Build history of the part. All positions in model axes, mm. Round coordinates to 2 decimals unless told otherwise and drop trailing zeros. Order: outer loops, then holes, each group sorted by start corner. A loop starts at its lowest first (then second) coordinate and runs counter-clockwise, first axis right, second up. Notation, with made-up numbers: M -33.75,5.25 L 8.25,5.25 A15 cw 8.25,9.25 Z; hole C 41.25,51.25 d6. An arc over 180 degrees is marked long. One line per item, written item: value. Start each with the question number.
Item 1: Band-saw the part on C-C, the plane x = 1.4. Write the cut outline in (y, z), then the cut area to 3 significant figures.
Item 2: Probe L1, parallel to Z at x = 1.15, y = 0; L2, parallel to Z at x = 1.3, y = 12.5; L3, parallel to Y at x = 2.15, z = 9.5. List the from-to ranges inside material, lowest first.
Item 3: Band-saw the part on A-A, the plane z = 0. Write the cut outline in (x, y), then the cut area to 3 significant figures.
Item 4: Pin check, flat tip, straight feed: pin 1 (1.5 mm diameter, centred on x = 0.5, z = 20.5, fed in from -Y). Stop position of the tip, or through.
Autodesk Inventor part; units mm, degrees
ref_plane "SW_HW_XY" through (-8.6667, 0, 0) normal (1, 0, 0) x (0, 0, -1)
ref_plane "SW_HW_YZ" through (-8.6667, 0, 0) normal (0, 0, -1) x (0, 1, 0)
ref_plane "SW_HW_ZX" through (-8.6667, 0, 0) normal (0, 1, 0) x (1, 0, 0)
sketch "Sketch_1" plane through (0, 0, 0) normal (0, 0, 1) x (1, 0, 0)
  line L0 (3.3333, 0) -> (0, 0)
  arc A0 (0, 20.8756) -> (0, 23.6244) centre (-2.6667, 22.25) ccw
  line L1 (0, 20.8756) -> (0, 18.1)
  arc A1 (0, 18.1) -> (0.6, 17.5) centre (0.6, 18.1) ccw
  line L2 (0.6, 17.5) -> (2.7333, 17.5)
  arc A2 (2.7333, 17.5) -> (3.3333, 18.1) centre (2.7333, 18.1) ccw
  line L3 (3.3333, 18.1) -> (3.3333, 25.4)
  arc A3 (3.3333, 25.4) -> (2.7333, 26) centre (2.7333, 25.4) ccw
  line L4 (2.7333, 26) -> (0.6, 26)
  arc A4 (0.6, 26) -> (0, 25.4) centre (0.6, 25.4) ccw
  line L5 (0, 25.4) -> (0, 23.6244)
revolve "Revolution1" add sketch "Sketch_1" angle 360 about axis through (3.3333, 0, 0) along (1, 0, 0)
ref_plane "SW_HW_XY" through (-8.6667, 0, 0) normal (1, 0, 0) x (0, 0, -1)
ref_plane "SW_HW_YZ" through (-8.6667, 0, 0) normal (0, 0, -1) x (0, 1, 0)
ref_plane "SW_HW_ZX" through (-8.6667, 0, 0) normal (0, 1, 0) x (1, 0, 0)
properties part number "51107 Shaft washer"
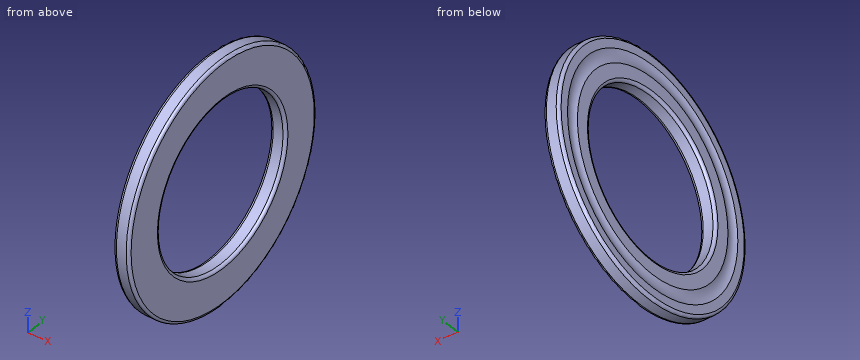
Output:
1. outline: C 0,0 d52; hole C 0,0 d35
1. area: 1,160 mm²
2. L1: z = -26 to -17.5, 17.5 to 26
2. L2: z = -22.8 to -12.25, 12.25 to 22.8
2. L3: y = -24.2 to -14.7, 14.7 to 24.2
3. outline: M 0,-25.4 A0.6 ccw 0.6,-26 L 2.73,-26 A0.6 ccw 3.33,-25.4 L 3.33,-18.1 A0.6 ccw 2.73,-17.5 L 0.6,-17.5 A0.6 ccw 0,-18.1 L 0,-20.88 A3 cw 0,-23.62 Z; M 0,18.1 A0.6 ccw 0.6,17.5 L 2.73,17.5 A0.6 ccw 3.33,18.1 L 3.33,25.4 A0.6 ccw 2.73,26 L 0.6,26 A0.6 ccw 0,25.4 L 0,23.62 A3 cw 0,20.88 Z
3. area: 54.8 mm²
4. pin 1: stops at y = -16.9
